Check sheet for the modelled part. Datum: model origin and axes. Units: mm. Round coordinates to 2 decimals unless told otherwise and drop trailing zeros. Write each loop counter-clockwise with the first axis right and the second up, starting at its lowest first coordinate (ties: lowest second). Pieces come first, ordered by that corner, then holes. Notation, with made-up numbers: M 33,68.25 L 63,68.25 A32 ccw 63,95.25 Z; hole C 55,18 d3. An arc over 180 degrees is marked long. Put each result on its own line as item: value.
Autodesk Inventor part; units mm, degrees
ref_plane "YZ Plane" through (0, 0, 0) normal (1, 0, 0) x (0, 1, 0)
ref_plane "XZ Plane" through (0, 0, 0) normal (0, 1, 0) x (-1, 0, 0)
ref_plane "XY Plane" through (0, 0, 0) normal (0, 0, 1) x (1, 0, 0)
sketch "Эскиз1" plane through (0, 0, 0) normal (0, 1, 0) x (-1, 0, 0)
  line L0 (-49.8359, -27.3218) -> (-34.1641, -27.3218)
  line L1 (-34.1641, -27.3218) -> (-31.3955, -24.5532)
  line L2 (-31.3955, -24.5532) -> (-31.3955, -24.5024)
  line L3 (-31.3955, -24.5024) -> (-34.1641, -21.7338)
  line L4 (-34.1641, -21.7338) -> (-34.1641, -18)
  line L5 (-34.1641, -18) -> (-30, -18)
  line L6 (-30, -18) -> (-30, -15)
  line L7 (-30, -15) -> (-54, -15)
  line L8 (-54, -15) -> (-54, -18)
  line L9 (-54, -18) -> (-49.8359, -18)
  line L10 (-49.8359, -18) -> (-49.8359, -21.7338)
  line L11 (-49.8359, -21.7338) -> (-52.6045, -24.5024)
  line L12 (-52.6045, -24.5024) -> (-52.6045, -24.5532)
  line L13 (-52.6045, -24.5532) -> (-49.8359, -27.3218)
  line L14 (-56.1832, -23.1562) -> (-23.3808, -23.1562) construction
  line L15 (-55.8733, -25.8994) -> (-24.0699, -25.8994) construction
  line L16 (-55.8733, -24.5278) -> (-24.0699, -24.5278) construction
  line L17 (-25.0606, -25.8994) -> (-25.0606, -24.5278) construction
  line L18 (-26.6052, -24.5278) -> (-26.6052, -23.1562) construction
  line L19 (-37.1641, -27.3218) -> (-38.6641, -24.3218)
  line L20 (-38.6641, -24.3218) -> (-45.3359, -24.3218)
  line L21 (-45.3359, -24.3218) -> (-46.8359, -27.3218)
  point P0 (0, 0)
  point P1 (-31.3955, -24.5278)
  dimension "d0" = 21.209
  dimension "d1" = 9.3218
  dimension "d2" = 15.6718
  dimension "d3" = 4.1656
  dimension "d4" = 2.7432
  dimension "d5" = 45
  dimension "d6" = 45
  dimension "d7" = 45
  dimension "d8" = 3
  dimension "d9" = 24
  dimension "d10" = 15
  dimension "d11" = 30
  dimension "d23" = 3
  dimension "d24" = 3
  dimension "d25" = 1.5
  dimension "d26" = 1.5
  dimension "d27" = 3
extrude "Выдавливание1" add sketch "Эскиз1" along normal mid plane 85
sketch "Эскиз2" plane through (54, -42.5, -18) normal (1, 0, 0) x (0, 0, -1)
  line L0 (9.3218, 85) -> (6.5532, 85)
  line L1 (6.3218, 85) -> (6.3218, 0)
  line L2 (6.5532, 0) -> (9.3218, 0)
  line L3 (9.3218, 85) -> (9.3218, 0)
  line L4 (9.3218, 0) -> (9.3218, 85)
  line L5 (9.3218, 80.2324) -> (6.3218, 80.2324)
  line L6 (9.3218, 75) -> (6.3218, 75)
  point P0 (-18, 42.5)
  dimension "d14" = 3
  dimension "d15" = 5.2324
  dimension "d16" = 10
extrude "Выдавливание2" cut sketch "Эскиз2" against normal through all
pattern_linear "Прямоуг.массив1" count 8 spacing 10 along (0, -1, 0) of "Выдавливание2"
equation "\"d24\" = d23"
equation "\"d26\" = d25"
properties part number "Rail_3DПЕЧАТЬ"
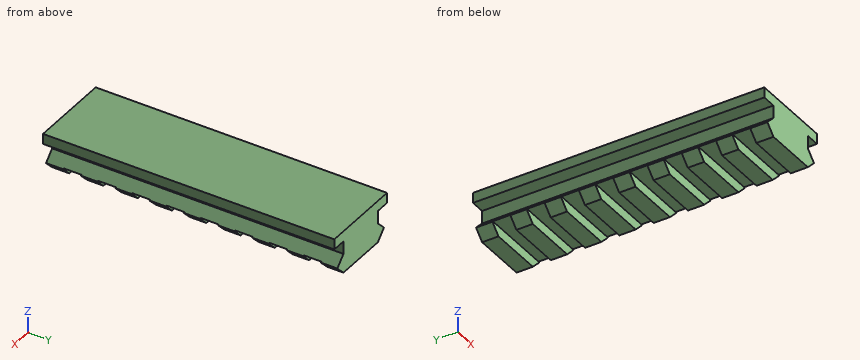
1. Cross-section at B-B (z = -20.75). Enter the section's corners in (x, y), then the cut area to 3 significant figures.
Computed values:
outline: M 34.16,-42.5 L 49.84,-42.5 L 49.84,42.5 L 34.16,42.5 Z
area: 1,330 mm2
2. Scan lines: probe 1 along Z at (x, y) = (37.25, 15); probe 2 along X at (y, z) = (34.5, -21); probe 3 along Z at (x, y) = (34, 11). Record each from-to range of solid material in increasing order.
Computed values:
probe 1: z = -24.32 to -15
probe 2: x = 34.16 to 49.84
probe 3: z = -27.16 to -21.9, -18 to -15
3. Cross-section at A-A (y = -16). Enter the section's corners in (x, z).
Computed values:
outline: M 30,-18 L 34.16,-18 L 34.16,-21.73 L 31.58,-24.32 L 52.42,-24.32 L 49.84,-21.73 L 49.84,-18 L 54,-18 L 54,-15 L 30,-15 Z
4. Depth check by flat-ended pin: pin 1 Ø2 at (y, z) = (0.5, -22) entering from -X; pin 2 Ø1 at (x, y) = (46, 23.5) entering from -Z; pin 3 Ø1 at (y, z) = (17.5, -24) entering from +X. Enter the tip coordinate at first touch or a pass-through.
Computed values:
pin 1: stops at x = 32.9
pin 2: stops at z = -24.32
pin 3: stops at x = 52.54
5. Cross-section at C-C (z = -26.25). Count the separate pieces of the cut face and the enclosed holes in it, then the cut area to 3 significant figures.
Computed values:
separate pieces: 9
enclosed holes: 0
area: 769 mm2
